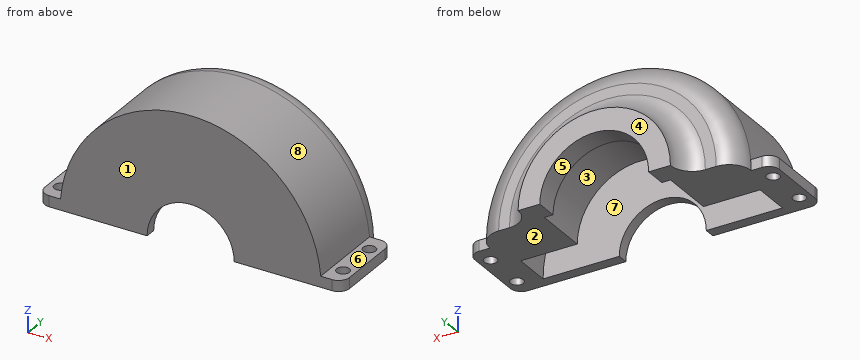
```python
from build123d import *

# Parameters (mm, degrees)
SKETCH1_R                = 25
SKETCH1_R_2              = 20
BOSS_EXTRUDE1_DEPTH      = 5
BOSS_EXTRUDE2_START      = -5
SKETCH2_R                = 60
SKETCH2_R_2              = 20
BOSS_EXTRUDE2_DEPTH      = 5
SKETCH3_R                = 60
SKETCH3_R_2              = 55
BOSS_EXTRUDE3_DEPTH      = 17
SKETCH4_R                = 60
SKETCH4_R_2              = 29
BOSS_EXTRUDE4_DEPTH      = 25
SKETCH5_R                = 35
SKETCH5_R_2              = 25
BOSS_EXTRUDE5_DEPTH      = 10
FILLET2_R                = 10
SKETCH6_W                = 10
SKETCH6_H                = 37
BOSS_EXTRUDE7_DEPTH      = 5
BOSS_EXTRUDE8_REACH      = 156.107
BOSS_EXTRUDE8_END_RADIUS = 60
SKETCH7_W                = 10
SKETCH7_H                = 37
M5_CLEARANCE_HOLE1_D     = 5.8
FILLET3_R                = 5


with BuildPart() as part:
    # Sketch1 → Boss-Extrude1 (new body)
    with BuildSketch(Plane(origin=(0, 0, 0), x_dir=(1, 0, 0), z_dir=(0, 1, 0))):
        with Locations(Location((0, 0, 0), (0, 0, 270))):
            Circle(SKETCH1_R)
        with Locations(Location((0, 0, 0), (0, 0, 270))):
            Circle(SKETCH1_R_2, mode=Mode.SUBTRACT)
    extrude(amount=BOSS_EXTRUDE1_DEPTH)

    # Sketch2 → Boss-Extrude2 (add)
    with BuildSketch(Plane(origin=(0, 5, 0), x_dir=(1, 0, 0), z_dir=(0, 1, 0)).offset(BOSS_EXTRUDE2_START)):
        with Locations(Location((0, 0, 0), (0, 0, 270))):
            Circle(SKETCH2_R)
        with Locations(Location((0, 0, 0), (0, 0, 270))):
            Circle(SKETCH2_R_2, mode=Mode.SUBTRACT)
    extrude(amount=BOSS_EXTRUDE2_DEPTH)

    # Sketch3 → Boss-Extrude3 (add)
    with BuildSketch(Plane(origin=(0, 5, 0), x_dir=(1, 0, 0), z_dir=(0, 1, 0))):
        with Locations(Location((0, 0, 0), (0, 0, 270))):
            Circle(SKETCH3_R)
        with Locations(Location((0, 0, 0), (0, 0, 270))):
            Circle(SKETCH3_R_2, mode=Mode.SUBTRACT)
    extrude(amount=BOSS_EXTRUDE3_DEPTH)

    # Sketch4 → Boss-Extrude4 (add)
    with BuildSketch(Plane(origin=(0, 22, 0), x_dir=(1, 0, 0), z_dir=(0, 1, 0))):
        with Locations(Location((0, 0, 0), (0, 0, 270))):
            Circle(SKETCH4_R)
        with Locations(Location((0, 0, 0), (0, 0, 270))):
            Circle(SKETCH4_R_2, mode=Mode.SUBTRACT)
    extrude(amount=BOSS_EXTRUDE4_DEPTH)

    # Sketch5 → Boss-Extrude5 (add)
    with BuildSketch(Plane(origin=(0, 47, 0), x_dir=(1, 0, 0), z_dir=(0, 1, 0))):
        with Locations(Location((0, 0, 0), (0, 0, 270))):
            Circle(SKETCH5_R)
        with Locations(Location((0, 0, 0), (0, 0, 270))):
            Circle(SKETCH5_R_2, mode=Mode.SUBTRACT)
    extrude(amount=BOSS_EXTRUDE5_DEPTH)

    # Fillet2
    fillet2_edges = [part.edges().sort_by_distance(p)[0] for p in [
        (0, 47, -60),
        (0, 47, -35),
    ]]
    fillet(fillet2_edges, radius=FILLET2_R - 0.0001)  # a hair under: the kernel refuses the full size



with BuildPart() as body_2:
    # Sketch6 → Boss-Extrude7 (new, symmetric)
    with BuildSketch(Plane.XY):
        with Locations((-65, 18.5)):
            Rectangle(SKETCH6_W, SKETCH6_H)
    extrude(amount=BOSS_EXTRUDE7_DEPTH, both=True)


with BuildPart() as part_1:
    add(part.part)

    add(body_2.part)  # Boss-Extrude8 merges body 2
    # Boss-Extrude8: up to this cylinder (the profile starts outside it)
    boss_extrude8_end = Plane(origin=(0, 18.5, 0), z_dir=(0, 1, 0)) * Cylinder(BOSS_EXTRUDE8_END_RADIUS, 433.214, mode=Mode.PRIVATE)
    # Sketch7 → Boss-Extrude8 (add, up to the surface)
    with BuildSketch(Plane.ZY.offset(70), mode=Mode.PRIVATE) as boss_extrude8_sk1:
        with Locations((0, 18.5)):
            Rectangle(SKETCH7_W, SKETCH7_H)
    boss_extrude8_tool1 = extrude(boss_extrude8_sk1.sketch, amount=-BOSS_EXTRUDE8_REACH, mode=Mode.PRIVATE) - boss_extrude8_end
    add(boss_extrude8_tool1.solids().sort_by_distance((-70, 18.5, 0))[0])

    # M5 Clearance Hole1 (through all)
    with Locations(Plane.XY.offset(5)):
        with Locations((-64.895651858, 8.5), (-64.895651858, 28.5)):
            Hole(M5_CLEARANCE_HOLE1_D / 2)

    # Fillet3
    fillet3_edges = [part_1.edges().sort_by_distance(p)[0] for p in [
        (-70, 37, 0),
        (-70, 0, 0),
    ]]
    fillet(fillet3_edges, radius=FILLET3_R)

    # Mirror1: part across plane


with BuildPart() as part_2:
    add(part_1.part)
    add(part_1.part.mirror(Plane(origin=(0, 0, 0), x_dir=(0, 0, 1), z_dir=(1, 0, 0))))


with BuildPart() as body_2_2:
    # Split1: the piece on the far side of the plane
    add(part_2.part)
    split(bisect_by=Plane.XY, keep=Keep.BOTTOM)


with BuildPart() as part_3:
    add(part_2.part)

    # Split1
    split(bisect_by=Plane.XY, keep=Keep.TOP)


solid = part_3.part
```
Verification items for the finished model (mm, model axes). Face numbers are marked on the shaded views. A direction names the side the tool comes from. Round coordinates to 2 decimals unless told otherwise and drop trailing zeros. Write each loop counter-clockwise with the first axis right and the second up, starting at its lowest first coordinate (ties: lowest second). Pieces come first, ordered by that corner, then holes.
1. Section check D-D on y = 50. Enter the section's corners in (x, z).
2. Gauge pin test, flat ends, axial feed: P1, Ø4.5, axis at x = 64.9, y = 8.5, coming from the +Z side; P2, Ø12, axis at y = 29, z = 16, coming from the +X side; P3, Ø8, axis at y = 15, z = 48, coming from the +X side; P4, Ø4, axis at y = 44, z = 35, coming from the +X side. Record the tip position at first contact, or that the pin passes through.
3. Scan lines: L1, parallel to Y at x = -47.5, z = 14; L2, parallel to X at y = 28, z = 3; L3, parallel to X at y = 33, z = 14. Record each from-to range of solid material in increasing order.
4. Draft check along Y on the marked faces 1, 2 and 3. Enter one of: +Y half, -Y half, draft (parallel to the pull), parting line (faces both ways), or undercut.
5. Access from +Z, -Z, +X, -X, +Y, -Y to the whole of each face (thin tool, end or side, straight path). Record for the marked faces 4, 5, 6, 7 and 8.
6. Section check A-A on y = 8.5. Enter the section's corners in (x, z), plus the area to 3 significant figures.
7. Section check C-C on y = 28.5. Enter the section's corners in (x, z), plus the area to 3 significant figures.
Answer:
1. outline: (-37.86, 0) - (-25, 0) arc R25 cw to (25, 0) - (37.86, 0) arc R37.86 ccw to start
2. P1: passes through
2. P2: stops at x = 59.16
2. P3: stops at x = 40.79
2. P4: stops at x = 47.65
3. L1: y = 0 to 5, 22 to 47
3. L2: x = -70 to -67.75, -62.04 to -28.84, 28.84 to 62.04, 67.75 to 70
3. L3: x = -58.34 to -25.4, 25.4 to 58.34
4. face 1: -Y half
4. face 2: draft
4. face 3: undercut
5. face 4: +Z, -Z, +X, -X, +Y
5. face 5: -Z, +Y
5. face 6: +Z, +X, +Y, -Y
5. face 7: -Z
5. face 8: +Z, +Y, -Y
6. outline: (-70, 0) - (-67.8, 0) - (-67.8, 5) - (-70, 5) - close; (-62, 0) - (-55, 0) arc R55 cw to (55, 0) - (62, 0) - (62, 5) - (59.79, 5) arc R60 ccw to (-59.79, 5) - (-62, 5) - close; (67.8, 0) - (70, 0) - (70, 5) - (67.8, 5) - close
6. area: 946 mm2
7. outline: (-70, 0) - (-67.8, 0) - (-67.8, 5) - (-70, 5) - close; (-62, 0) - (-29, 0) arc R29 cw to (29, 0) - (62, 0) - (62, 5) - (59.79, 5) arc R60 ccw to (-59.79, 5) - (-62, 5) - close; (67.8, 0) - (70, 0) - (70, 5) - (67.8, 5) - close
7. area: 4,380 mm2
